Geometry check sheet. Reference: the model listing, model coordinates, mm. Face numbers are marked on the shaded views. A direction names the side the tool comes from. Give positions to 0.01 mm unless a question says otherwise; leave off trailing zeros. Order: outer loops, then holes, each group sorted by start corner. A loop starts at its lowest first (then second) coordinate and runs counter-clockwise, first axis right, second up.
```python
from build123d import *

# Parameters (mm, degrees)
SKETCH1_R           = 0.5969
BOSS_EXTRUDE1_DEPTH = 0.889


with BuildPart() as part:
    # Sketch1 → Boss-Extrude1 (new body)
    with BuildSketch(Plane.XY):
        with BuildLine():
            Line((-5.68137307, -3.048), (-2.981745785, -3.048))
            ThreePointArc((-2.981745785, -3.048), (-2.321834428, -3.429), (-2.321834428, -4.191))
            Line((-2.321834428, -4.191), (-3.275039722, -5.842))
            ThreePointArc((-3.275039722, -5.842), (-3.775058057, -6.206035718), (-4.38041724, -6.079226415))
            ThreePointArc((-4.38041724, -6.079226415), (0, 7.493), (4.38041724, -6.079226415))
            ThreePointArc((4.38041724, -6.079226415), (3.775058057, -6.206035718), (3.275039722, -5.842))
            Line((3.275039722, -5.842), (2.321834428, -4.191))
            ThreePointArc((2.321834428, -4.191), (2.321834428, -3.429), (2.981745785, -3.048))
            Line((2.981745785, -3.048), (5.68137307, -3.048))
            ThreePointArc((5.68137307, -3.048), (5.968179451, -2.95929238), (6.154820826, -2.72415))
            ThreePointArc((6.154820826, -2.72415), (0, 6.2738), (-6.154820826, -2.72415))
            ThreePointArc((-6.154820826, -2.72415), (-5.968179451, -2.95929238), (-5.68137307, -3.048))
        make_face()
        with Locations((-3.6195, -4.318)):
            Circle(SKETCH1_R, mode=Mode.SUBTRACT)
        with Locations(Location((3.6195, -4.318, 0), (0, 0, 180))):
            Circle(SKETCH1_R, mode=Mode.SUBTRACT)
    extrude(amount=BOSS_EXTRUDE1_DEPTH)


solid = part.part
```
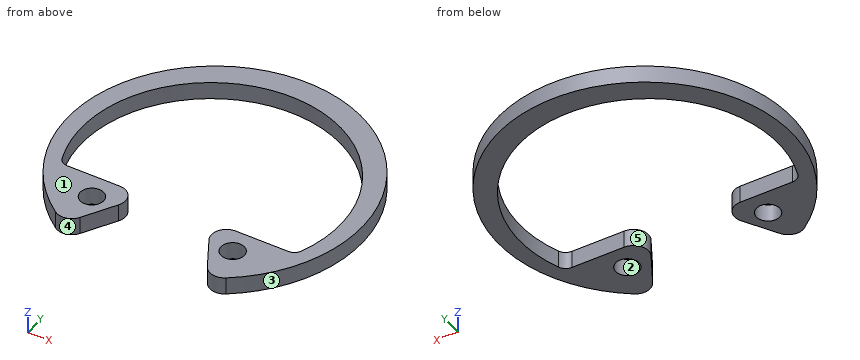
Q1. Cross-section at D-D, the plane x = 0. Record the boundary of the cut face in (y, z), and give its area (3 significant figures).
Q2. Thickness scan on L1, parallel to X at y = -4.25, z = 0.5; L2, parallel to Y at x = 3.5, z = 0.7; L3, parallel to Y at x = 0, z = 0.7. Record the ranges inside material, lowest first.
Q3. Cross-section at A-A, the plane y = 2.25. Record the boundary of the cut face in (x, z), and give its area (3 significant figures).
Q4. Release check for a two-part mould opening along X. For the marked faces 1, 2 and 3 record: pulls with the +X half, pulls with the -X half, needs draft (parallel to the pull), parting line crosses it, or undercut.
Q5. Cross-section at C-C, the plane z = 0.25. Record the boundary of the cut face in (x, y).
Q6. Cross-section at B-B, the plane x = -3.75. Record the boundary of the cut face in (y, z).
Q7. Access from +Z, -Z, +X, -X, +Y, -Y to the whole of each face (thin tool, end or side, straight path). Record for the marked faces 4 and 5.
Answers follow:
1. outline: (6.27, 0) - (7.49, 0) - (7.49, 0.89) - (6.27, 0.89) - close
1. area: 1.08 mm2
2. L1: x = -6.17 to -4.21, -3.03 to -2.36, 2.36 to 3.03, 4.21 to 6.17
2. L2: y = -6.09 to -4.9, -3.73 to -3.05, 5.27 to 6.63
2. L3: y = 6.27 to 7.49
3. outline: (-7.15, 0) - (-6.08, 0) - (-6.08, 0.89) - (-7.15, 0.89) - close; (6.08, 0) - (7.15, 0) - (7.15, 0.89) - (6.08, 0.89) - close
3. area: 1.90 mm2
4. face 1: needs draft
4. face 2: undercut
4. face 3: parting line crosses it
5. outline: (-6.15, -2.72) arc R6.6 cw (long way) to (6.15, -2.72) arc R0.51 cw to (5.68, -3.05) - (2.98, -3.05) arc R0.76 ccw to (2.32, -4.19) - (3.28, -5.84) arc R0.76 ccw to (4.38, -6.08) arc R7.49 ccw (long way) to (-4.38, -6.08) arc R0.76 ccw to (-3.28, -5.84) - (-2.32, -4.19) arc R0.76 ccw to (-2.98, -3.05) - (-5.68, -3.05) arc R0.51 cw to start; hole circle Ø1.19 at (-3.62, -4.32); hole circle Ø1.19 at (3.62, -4.32)
6. outline: (-6.2, 0) - (-4.9, 0) - (-4.9, 0.89) - (-6.2, 0.89) - close; (-3.74, 0) - (-3.05, 0) - (-3.05, 0.89) - (-3.74, 0.89) - close; (5.11, 0) - (6.49, 0) - (6.49, 0.89) - (5.11, 0.89) - close
7. face 4: +Z, -Z, -Y
7. face 5: +Z, -Z
